Design review of the part built by this model. Coordinates are the model's own, in mm. A direction names the side the tool comes from. Round coordinates to 2 decimals unless told otherwise and drop trailing zeros. Write each loop counter-clockwise with the first axis right and the second up, starting at its lowest first coordinate (ties: lowest second). Pieces come first, ordered by that corner, then holes. Notation, with made-up numbers: M 12.25,29 L 40.25,29 A24 ccw 40.25,51 Z; hole C -15,88.5 d5. An arc over 180 degrees is marked long. Use CSV: the item, a comma, the result in double quotes.
from build123d import *

# Parameters (mm, degrees)
SKETCH_1_R          = 1.357591064
SKETCH_1_R_2        = 3.543825796
SKETCH_1_W          = 5.3728
SKETCH_1_H          = 3.0001
SKETCH_1_W_2        = 7.9992
EXTRUDE_1_DEPTH     = 3
SKETCH_2_R          = 1.6
CUT_EXTRUDE_1_DEPTH = 57.708942736


with BuildPart() as part:
    # 草图1 → 凸台-拉伸1 (new body)
    with BuildSketch(Plane.XY.offset(3)):
        with BuildLine():
            Line((30.618171933, 12), (-49.343510787, 12))
            ThreePointArc((-49.343510787, 12), (-55.343510787, 6), (-49.343510787, 0))
            Line((-49.343510787, 0), (30.618171933, 0))
            ThreePointArc((30.618171933, 0), (36.618171933, 6), (30.618171933, 12))
        make_face()
        with Locations(Location((30.611606698, 6.0001, 0), (0, 0, 180))):
            Circle(SKETCH_1_R, mode=Mode.SUBTRACT)
        with Locations(Location((-13.375343302, 6.0002, 0), (0, 0, 180))):
            Circle(SKETCH_1_R, mode=Mode.SUBTRACT)
        with Locations(Location((-49.343510787, 6, 0), (0, 0, 180))):
            Circle(SKETCH_1_R_2, mode=Mode.SUBTRACT)
        with Locations((-23.691393302, 5.99945)):
            Rectangle(SKETCH_1_W, SKETCH_1_H, mode=Mode.SUBTRACT)
        with Locations((16.621706698, 5.99945)):
            Rectangle(SKETCH_1_W_2, SKETCH_1_H, mode=Mode.SUBTRACT)
        with BuildLine():
            Line((-34.404739086, 5.1001), (-39.352347519, 5.1001))
            ThreePointArc((-39.352347519, 5.1001), (-40.269423986, 6.017176468), (-39.352347519, 6.934252935))
            Line((-39.352347519, 6.934252935), (-34.404739086, 6.934252935))
            ThreePointArc((-34.404739086, 6.934252935), (-33.487662618, 6.017176468), (-34.404739086, 5.1001))
        make_face(mode=Mode.SUBTRACT)
    extrude(amount=-EXTRUDE_1_DEPTH)

    # 草图2 → 切除-拉伸1 (cut, through all)
    with BuildSketch(Plane.XY.offset(3)):
        with Locations((-13.375343302, 6.0002)):
            Circle(SKETCH_2_R)
    extrude(amount=-CUT_EXTRUDE_1_DEPTH, mode=Mode.SUBTRACT)


solid = part.part
1) Add section B-B on z = 1.6. Write out the cut boundary in (x, y) (1 decimal), then the cut area to 3 significant figures.
Answers:
outline,"M -49.3,0 L 30.6,0 A6 ccw 30.6,12 L -49.3,12 A6 ccw Z; hole C -49.3,6 d7.1; hole M -39.4,5.1 L -34.4,5.1 A0.9 ccw -34.4,6.9 L -39.4,6.9 A0.9 ccw Z; hole M -26.4,4.5 L -21,4.5 L -21,7.5 L -26.4,7.5 Z; hole C -13.4,6 d3.2; hole M 12.6,4.5 L 20.6,4.5 L 20.6,7.5 L 12.6,7.5 Z; hole C 30.6,6 d2.7"
area,"968 mm²"
2) The part is to be moulded in two halves that separate along X. For faces 3 (the face through (-55.342, 6.132, 1.521)), 4 (the face through (-9, 12, 2)), 5 (the face through (-33.488, 6.037, 1.521)), say which applies: released by +X, released by -X, zero draft, split by the parting line, or undercut.
Answers:
face 3,"released by -X"
face 4,"zero draft"
face 5,"undercut"
3) For pin 1 Ø5.5 at (x, y) = (-49.34, 6) entering from -Z, flat-tipped, find the tip position at first contact; note if it passes through.
Answers:
pin 1,"through"
4) Add section A-A on x = -37. Write out the cut boundary in (y, z).
Answers:
outline,"M 0,0 L 5.1,0 L 5.1,3 L 0,3 Z; M 6.93,0 L 12,0 L 12,3 L 6.93,3 Z"
5) Wall thickness on line 1 along Y through (x, z) = (18, 2.3); line 2 along Y through (x, z) = (-38, 1.15); line 3 along X through (y, z) = (9.25, 2.8): over which ranges is each line inside the solid? List them lowest first. Write a range as [from, to].
Answers:
line 1,"[0, 4.5], [7.5, 12]"
line 2,"[0, 5.1], [6.93, 12]"
line 3,"[-54.39, -50.76], [-47.93, 35.66]"
6) Machinability: for faces 1 (the face through (12.622, 6, 2)), 2 (the face through (-10, 6, 0)), which of the approach directions +Z, -Z, +X, -X, +Y, -Y give a long, thin tool a straight path to every point of the face, cutting with its end or side? Answer none if there is none.
Answers:
face 1,"+Z, -Z"
face 2,"-Z, +X, -X, +Y, -Y"
